Answer from the drawing. Dimensions are ordinates in mm from the lowest x, y and z of the part. Give positions to 0.01 mm unless a question says otherwise; leave off trailing zeros. Loops run counter-clockwise (first coordinate to the right, second up) from the corner with the lowest first, then second, coordinate; pieces in that order, holes last. Notation, with made-up numbers: (89, -31.75) - (145, -31.75) arc R23 ccw to (145, -16.75) - close; hole circle Ø3 at (6, 87). An arc over 180 degrees is marked (long way). Answer as CSV lines item,"result". Start each with the question number.
1) A cutting plane is placed at A-A (y = 5). Determine the outline of the cut face in (x, z).
2) A cutting plane is placed at D-D (y = 1.5). Determine the outline of the cut face in (x, z).
3) A cutting plane is placed at C-C (z = 4). Determine the outline of the cut face in (x, y), and give its area (3 significant figures).
4) Find the intervals of material crossed by line 1 along Z through (x, y) = (29.5, 7.5); line 2 along X through (y, z) = (4.25, 19); line 3 along Z through (x, y) = (9.5, 4.75), in increasing order.
5) A cutting plane is placed at B-B (x = 17). Determine the outline of the cut face in (y, z).
6) Flat-ended cylindrical pins translate along their axes: pin 1 (18 mm diameter, centred on x = 17, z = 17, fed in from +Y); pin 2 (1.1 mm diameter, centred on x = 18.5, y = 6, fed in from +Z); pin 3 (2 mm diameter, centred on x = 16, z = 16, fed in from +Y). Find the tip coordinate at first contact, or state that the pin passes through.
7) For a pull along Z with two mould halves and no side action, classify the marked faces 1, 2, 3 and 4 as pulls with the +Z half, pulls with the -Z half, needs draft (parallel to the pull), parting line crosses it, or undercut.
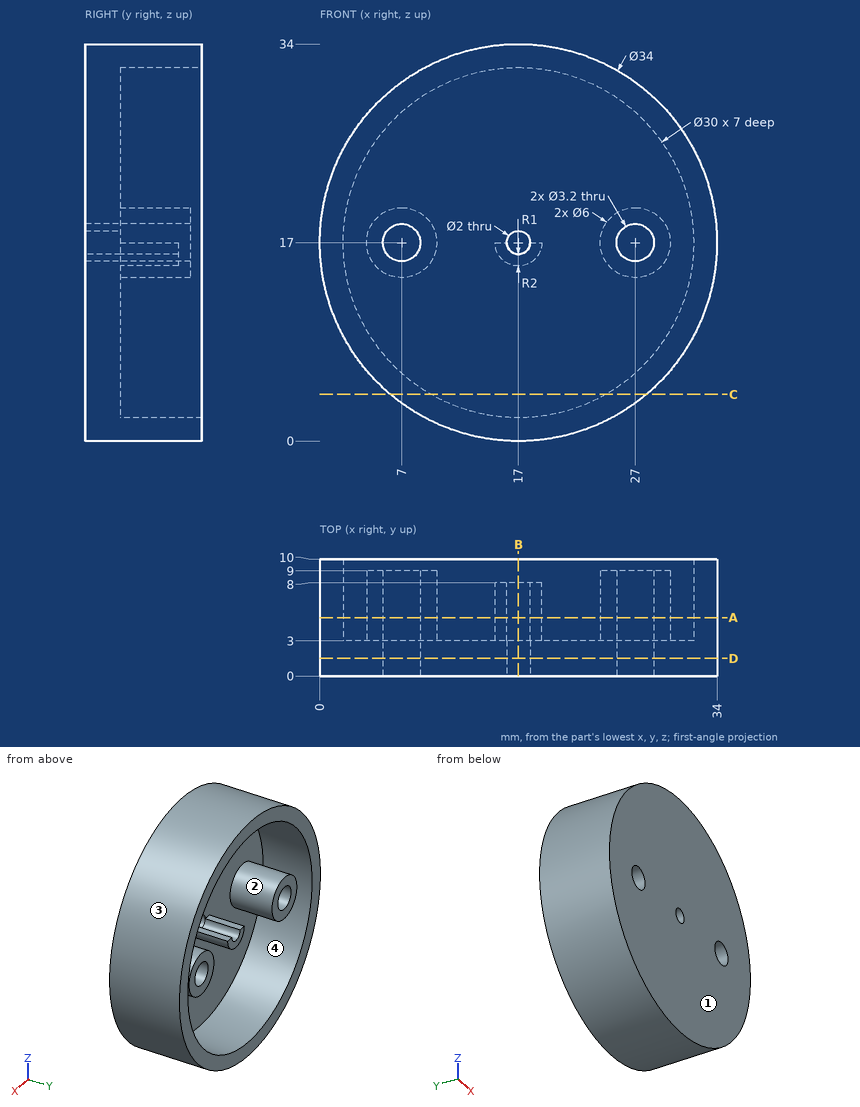
Ans:
1,outline,"circle Ø34 at (17, 17); circle Ø6 at (7, 17); (15, 17) arc R2 ccw to (19, 17) - (18, 17) arc R1 cw to (16, 17) - close; circle Ø6 at (27, 17); hole circle Ø30 at (17, 17); hole circle Ø3.2 at (7, 17); hole circle Ø3.2 at (27, 17)"
2,outline,"circle Ø34 at (17, 17); hole circle Ø3.2 at (7, 17); hole circle Ø2 at (17, 17); hole circle Ø3.2 at (27, 17)"
3,outline,"(6.05, 0) - (27.95, 0) - (27.95, 10) - (24.48, 10) - (24.48, 3) - (9.52, 3) - (9.52, 10) - (6.05, 10) - close"
3,area,"114 mm2"
4,line 1,"5.48 to 8.71, 15.34 to 18.66, 25.29 to 28.52"
4,line 2,"0.12 to 2.13, 4.76 to 9.24, 24.76 to 29.24, 31.87 to 33.88"
4,line 3,"1.74 to 4.01, 15.34 to 18.66, 29.99 to 32.26"
5,outline,"(0, 0) - (10, 0) - (10, 2) - (3, 2) - (3, 15) - (8, 15) - (8, 16) - (0, 16) - close; (0, 18) - (3, 18) - (3, 32) - (10, 32) - (10, 34) - (0, 34) - close"
6,pin 1,"y = 9"
6,pin 2,"z = 33.97"
6,pin 3,"y = 8"
7,face 1,"needs draft"
7,face 2,"undercut"
7,face 3,"parting line crosses it"
7,face 4,"undercut"
